from build123d import *

# Parameters (mm, degrees)
CUT_EXTRUDE1_START = 8.999999866
CUT_EXTRUDE1_DEPTH = 2.000000134


with BuildPart() as part:
    # Sketch2 → Revolve1 (revolve)
    with BuildSketch(Plane(origin=(0, 0, 0), x_dir=(0, 0, -1), z_dir=(1, 0, 0)), mode=Mode.PRIVATE) as revolve1_sk:
        with BuildLine():
            Line((10, 0), (10, 0.6))
            Line((10, 0.6), (9.6, 1))
            Line((9.6, 1), (-8, 1))
            Line((-8, 1), (-8, 1.8))
            ThreePointArc((-8, 1.8), (-8.029289322, 1.870710678), (-8.1, 1.9))
            Line((-8.1, 1.9), (-9.9, 1.9))
            ThreePointArc((-9.9, 1.9), (-9.970710678, 1.870710678), (-10, 1.8))
            Line((-10, 1.8), (-10, 0.75))
            Line((-10, 0.75), (-9, 0.75))
            Line((-9, 0.75), (-8.566987298, 0))
            Line((-8.566987298, 0), (10, 0))
        make_face()
    revolve(revolve1_sk.sketch.rotate(Axis((0, 0, -10), (0, 0, 1)), 90), axis=Axis((0, 0, -10), (0, 0, 1)))

    # Cut-Extrude1: read off the stored shape, not the designer's step
    # Cut-Extrude1 outline → Cut-Extrude1 (cut)
    with BuildSketch(Plane.XY.offset(CUT_EXTRUDE1_START)):
        with BuildLine():
            Line((0.375000005, 0.64951905), (0, 0.866025404))
            Line((0, 0.866025404), (-0.374999989, 0.649519059))
            ThreePointArc((-0.374999989, 0.649519059), (9e-09, 0.75), (0.375000005, 0.64951905))
        make_face()
        with BuildLine():
            ThreePointArc((-0.75, 0), (-0.64951905, 0.375000005), (-0.374999989, 0.649519059))
            Line((-0.374999989, 0.649519059), (-0.75, 0.433012702))
            Line((-0.75, 0.433012702), (-0.75, 0))
        make_face()
        with BuildLine():
            Line((0.75, 0.433012702), (0.375000005, 0.64951905))
            ThreePointArc((0.375000005, 0.64951905), (0.649519054, 0.374999997), (0.75, 0))
            Line((0.75, 0), (0.75, 0.433012702))
        make_face()
        with BuildLine():
            ThreePointArc((-0.375000002, -0.649519052), (-0.649519053, -0.374999999), (-0.75, 0))
            Line((-0.75, 0), (-0.75, -0.433012702))
            Line((-0.75, -0.433012702), (-0.375000002, -0.649519052))
        make_face()
        with BuildLine():
            Line((0.75, -0.433012702), (0.75, 0))
            ThreePointArc((0.75, 0), (0.649519051, -0.375000003), (0.374999994, -0.649519056))
            Line((0.374999994, -0.649519056), (0.75, -0.433012702))
        make_face()
        with BuildLine():
            ThreePointArc((0.374999994, -0.649519056), (-5e-09, -0.75), (-0.375000002, -0.649519052))
            Line((-0.375000002, -0.649519052), (0, -0.866025404))
            Line((0, -0.866025404), (0.374999994, -0.649519056))
        make_face()
    extrude(amount=CUT_EXTRUDE1_DEPTH, mode=Mode.SUBTRACT)

    # Cut-Extrude1 2 outline → Cut-Extrude1 2 (revolve)
    with BuildSketch(Plane.XZ):
        Polygon((0.866025458, 9.066987329), (0.749999942, 8.999999966), (0.866025404, 8.999999866), align=None)
    revolve(axis=Axis((0, 0, 0), (0, 0, 1)))

    # Cut-Extrude2 cone 1 section (on through the dimple's axis) → Cut-Extrude2 (revolve, cut)
    with BuildSketch(Plane(origin=(0, 0, 10), x_dir=(0, -1, 0), z_dir=(1, 0, 0))):
        Polygon((0, 0), (1.116025404, 0), (0, 0.644337567), align=None)
    revolve(axis=Axis((0, 0, 10), (0, 0, -1)), mode=Mode.SUBTRACT)


solid = part.part
Could you check a few things on this model? Use its own coordinates, in mm. A direction names the side the tool comes from. Round coordinates to 2 decimals unless told otherwise and drop trailing zeros. Order: outer loops, then holes, each group sorted by start corner. A loop starts at its lowest first (then second) coordinate and runs counter-clockwise, first axis right, second up.
Q1. I'm going to push a flat-ended pin straight in: P1, Ø1.5, axis at y = 1, z = -2, coming from the +X side. Where does the tip first touch, or does it pass through?
Geometry says:
P1: stops at x = 0.97
Q2. Imagine slicing it at A-A, the plane z = -2. List the corners of the cut face in (x, y) for me.
Geometry says:
outline: circle Ø2 at (0, 0)
Q3. Which directions (+Z, -Z, +X, -X, +Y, -Y) give clear straight access to the entire face, cutting with the end or side of a thin tool? Please do faces 1 (the face through (0.75, 0, 9.4)), 2 (the face through (0, 0, -10)), 3 (the face through (1, 1, 8)).
Geometry says:
face 1: +Z
face 2: -Z, +X, -X, +Y, -Y
face 3: -Z
Q4. Please list where these lines run through material, in increasing order: probe 1 along Z at (x, y) = (0.5, -1.1); probe 2 along Y at (x, z) = (-0.8, -8); probe 3 along X at (y, z) = (-0.1, 4.5).
Geometry says:
probe 1: z = 8 to 10
probe 2: y = -0.6 to 0.6
probe 3: x = -0.99 to 0.99
Q5. Thinking about a two-plate mould opening in Y: for faces 4 (the face through (1, 1, 10)), 5 (the face through (-1.812, -0.571, 9.013)), 6 (the face through (-0.75, 0, 9.4)), which applies, released by +Y, released by -Y, zero draft, split by the parting line, or undercut?
Geometry says:
face 4: zero draft
face 5: split by the parting line
face 6: undercut
